```python
from build123d import *

# Parameters (mm, degrees)
F1_DEPTH       = 22.5
F2_W           = 45
F2_H           = 15.3
F3_DEPTH       = 3
F5_D           = 3
F5_DEPTH       = 4
F5_CSINK_D     = 4
F5_CSINK_ANGLE = 90
F5_TIP         = 0.9012909285


with BuildPart() as f1:
    # F0 (on Right) → F1 (new body, symmetric)
    with BuildSketch(Plane.YZ):
        Polygon((7.65, 0), (7.65, 11.2), (1.175, 11.2), (1.175, 8.2), (2.65, 8.2), (2.65, 6), (0, 6), (0, 0), align=None)
        Polygon((-7.65, 0), (0, 0), (0, 6), (-2.65, 6), (-2.65, 8.2), (-1.175, 8.2), (-1.175, 11.2), (-7.65, 11.2), align=None)
    extrude(amount=F1_DEPTH, both=True)

    # F2 (on face) → F3 (join)
    with BuildSketch(Plane(origin=(0, 0, 0), x_dir=(1, 0, 0), z_dir=(0, 0, -1))):
        with BuildLine():
            Line((22.5, 7.65), (22.5, -7.65))
            Line((22.5, -7.65), (26.5, -7.65))
            ThreePointArc((26.5, -7.65), (34.15, 0), (26.5, 7.65))
            Line((26.5, 7.65), (22.5, 7.65))
        make_face()
        Rectangle(F2_W, F2_H)
        with BuildLine():
            Line((-26.5, -7.65), (-22.5, -7.65))
            Line((-22.5, -7.65), (-22.5, 7.65))
            Line((-22.5, 7.65), (-26.5, 7.65))
            ThreePointArc((-26.5, 7.65), (-34.15, 0), (-26.5, -7.65))
        make_face()
    extrude(amount=-F3_DEPTH)

    # F5
    with Locations(Plane.XY.offset(3)):
        with Locations((26.5, 0), (-26.5, 0)):
            CounterSinkHole(F5_D / 2, F5_CSINK_D / 2, depth=F5_DEPTH, counter_sink_angle=F5_CSINK_ANGLE)
            with Locations((0, 0, -(F5_DEPTH + F5_TIP / 2))):  # 118° drill point
                Cone(0, F5_D / 2, F5_TIP, mode=Mode.SUBTRACT)


solid = f1.part
```
Can you work these out from the model? Positions are in its coordinate system, mm. A direction names the side the tool comes from. Coordinates: 2 decimals unless noted, no trailing zeros. Loops run counter-clockwise (first coordinate to the right, second up) from the corner with the lowest first, then second, coordinate; pieces in that order, holes last.
1) Thinking about a two-plate mould opening in X: for faces 5 (the cylindrical face through (-34.15, -0.17, 1.48)), 6 (the flat face through (0, 2.65, 7)), 7 (the cylindrical face through (28, 0, 1)), which applies, pulls with the +X half, pulls with the -X half, needs draft (parallel to the pull), parting line crosses it, or undercut?
2) For pin 1 (6 mm diameter, centred on x = 5, y = 1, fed in from +Z); pin 2 (1 mm diameter, centred on y = -5, z = 6, fed in from +X); pin 3 (4 mm diameter, centred on y = -0.5, z = 5.5, fed in from -X); pin 4 (6 mm diameter, centred on x = -30.5, y = 2.5, fed in from +Z), each with a flat end and sliding along its axis, tell me the tip position at first contact or that it passes through.
3) Imagine slicing it at A-A on y = 0. List the corners of the cut face in (x, z) for me.
4) Imagine slicing it at B-B on z = 6.75. List the corners of the cut face in (x, y) for me.
5) I need wall thicknesses on probe 1 along Y at (x, z) = (-26.5, 1.9); probe 2 along X at (y, z) = (0, 1.5); probe 3 along X at (y, z) = (-1.75, 9.25). Which ranges of each line are inside material? Lowest first, please.
6) Imagine slicing it at D-D on y = 6. List the corners of the cut face in (x, z) for me, plus the area to 3 significant figures.
7) Imagine slicing it at C-C on x = 12. List the corners of the cut face in (y, z) for me (3 decimals), plus the area to 3 significant figures.
8) Which directions (+Z, -Z, +X, -X, +Y, -Y) give clear straight access to the entire face, cutting with the end or side of a thin tool? Please do faces 1 (the flat face through (-22.5, 0, 5)), 2 (the flat face through (0, -1.175, 10)), 3 (the flat face through (0, -2.65, 7)), 4 (the flat face through (22.5, 0, 5)).
Completed:
1. face 5: pulls with the -X half
1. face 6: needs draft
1. face 7: undercut
2. pin 1: stops at z = 11.2
2. pin 2: stops at x = 22.5
2. pin 3: stops at x = -22.5
2. pin 4: stops at z = 3
3. outline: (-34.15, 0) - (-28, 0) - (-28, 2.5) - (-28.5, 3) - (-34.15, 3) - close; (-25, 0) - (25, 0) - (25, 2.5) - (24.5, 3) - (22.5, 3) - (22.5, 6) - (-22.5, 6) - (-22.5, 3) - (-24.5, 3) - (-25, 2.5) - close; (28, 0) - (34.15, 0) - (34.15, 3) - (28.5, 3) - (28, 2.5) - close
4. outline: (-22.5, -7.65) - (22.5, -7.65) - (22.5, -2.65) - (-22.5, -2.65) - close; (-22.5, 2.65) - (22.5, 2.65) - (22.5, 7.65) - (-22.5, 7.65) - close
5. probe 1: y = -7.65 to -1.5, 1.5 to 7.65
5. probe 2: x = -34.15 to -28, -25 to 25, 28 to 34.15
5. probe 3: x = -22.5 to 22.5
6. outline: (-31.25, 0) - (31.25, 0) - (31.25, 3) - (22.5, 3) - (22.5, 11.2) - (-22.5, 11.2) - (-22.5, 3) - (-31.25, 3) - close
6. area: 556 mm2
7. outline: (-7.65, 0) - (7.65, 0) - (7.65, 11.2) - (1.175, 11.2) - (1.175, 8.2) - (2.65, 8.2) - (2.65, 6) - (-2.65, 6) - (-2.65, 8.2) - (-1.175, 8.2) - (-1.175, 11.2) - (-7.65, 11.2) - close
7. area: 153 mm2
8. face 1: +Z, -X, +Y, -Y
8. face 2: +Z, +X, -X
8. face 3: +X, -X
8. face 4: +Z, +X, +Y, -Y
